Part model, mm, in its own coordinate system. A direction names the side the tool comes from. Round coordinates to 2 decimals unless told otherwise and drop trailing zeros. Return JSON: item names as keys, results as strings. Group by question number.
Item 1: Two-plate mould, pull along Y, no slides. Class faces 1 (the face through (0, 0, 0)), 2 (the face through (-1.625, 5.99, 12.166)), 3 (the face through (-6.73, 14.59, 13.97)), 4 (the face through (-3.042, -5.172, 13.944)): released by +Y, released by -Y, zero draft, split by the parting line, or undercut.
Item 2: Tool access for faces 5 (the face through (0, 0, 19)), 6 (the face through (3.042, 5.172, 13.944)), 7 (the face through (-1, 2, 18)): list every direction of +Z, -Z, +X, -X, +Y, -Y with a clear straight run to the whole face (end or side of a thin tool).
Item 3: Drop flat-ended pins along their axis: pin 1 (7.5 mm diameter, centred on y = -1.5, z = 14, fed in from -X); pin 2 (1.2 mm diameter, centred on x = 0.5, y = -0.5, fed in from +Z); pin 3 (1 mm diameter, centred on x = 5.5, z = 9, fed in from -Y); pin 4 (1.5 mm diameter, centred on x = -7.5, z = 26.5, fed in from -Y). Give the stop position or say it passes through.
Item 4: Probe probe 1 along Y at (x, z) = (0, 23.25); probe 2 along Z at (x, y) = (0.5, -0.75); probe 3 along Z at (x, y) = (-3, -1.75). List the from-to ranges inside material, lowest first.
Item 5: Saw through at A-A on x = -3.25. State how many separate pieces and enclosed holes the cut face has, and give its area (3 significant figures).
```python
from build123d import *

# Parameters (mm, degrees)
SKETCH_1_R          = 2.5
EXTRUDE_1_DEPTH     = 10
EXTRUDE_2_DEPTH     = 8
SKETCH_3_R          = 2
EXTRUDE_3_DEPTH     = 1
SKETCH_5_R          = 0.75
CUT_EXTRUDE_1_DEPTH = 15
SKETCH_6_R          = 2.25
EXTRUDE_4_DEPTH     = 10
SKETCH_7_R          = 1.25
CUT_EXTRUDE_2_DEPTH = 22


with BuildPart() as part:
    # 草图1 → 凸台-拉伸1 (new body)
    with BuildSketch(Plane.XY):
        Circle(SKETCH_1_R)
    extrude(amount=EXTRUDE_1_DEPTH)

    # 草图2 → 凸台-拉伸2 (add)
    with BuildSketch(Plane.XY.offset(10)):
        Polygon((6, 3.464101615), (0, 6.92820323), (-6, 3.464101615), (-6, -3.464101615), (0, -6.92820323), (6, -3.464101615), align=None)
    extrude(amount=EXTRUDE_2_DEPTH)

    # 草图3 → 凸台-拉伸3 (add)
    with BuildSketch(Plane.XY.offset(18)):
        Circle(SKETCH_3_R)
    extrude(amount=EXTRUDE_3_DEPTH)

    # 草图4 → 旋转1 (revolve)
    with BuildSketch(Plane(origin=(0, 0, 0), x_dir=(1, 0, 0), z_dir=(0, 1, 0)), mode=Mode.PRIVATE) as revolve_1_sk:
        Polygon((0, -19), (7.5, -19), (7.5, -27), (1.664204883, -31.183358747), (2.5, -34), (0, -34), align=None)
    revolve(revolve_1_sk.sketch.rotate(Axis((0, 0, 19), (0, 0, 1)), 180), axis=Axis((0, 0, 19), (0, 0, 1)))

    # 草图5 → 切除-拉伸1 (cut)
    with BuildSketch(Plane.XY.offset(34)):
        Circle(SKETCH_5_R)
    extrude(amount=-CUT_EXTRUDE_1_DEPTH, mode=Mode.SUBTRACT)

    # 草图6 → 凸台-拉伸4 (add)
    with BuildSketch(Plane(origin=(-3, 5.196152423, 0), x_dir=(0.8660254037844388, 0.49999999999999983, 0), z_dir=(-0.4999999999999998, 0.8660254037844387, 0))):
        with Locations((0, -14)):
            Circle(SKETCH_6_R)
    extrude(amount=EXTRUDE_4_DEPTH)

    # 草图7 → 切除-拉伸2 (cut)
    with BuildSketch(Plane(origin=(-8, 13.856406461, 0), x_dir=(0.8660254037844387, 0.49999999999999994, 0), z_dir=(-0.4999999999999999, 0.8660254037844386, 0))):
        with Locations(Location((0, -14, 0), (0, 0, 180))):
            Circle(SKETCH_7_R)
    extrude(amount=-CUT_EXTRUDE_2_DEPTH, mode=Mode.SUBTRACT)


solid = part.part
```
Filled in:
{
 "1": {"face 1": "zero draft", "face 2": "undercut", "face 3": "released by +Y", "face 4": "released by -Y"},
 "2": {"face 5": "+Z", "face 6": "-Z, +X, +Y", "face 7": "none"},
 "3": {"pin 1": "stops at x = -6", "pin 2": "stops at z = 34", "pin 3": "passes through", "pin 4": "stops at y = -3.27"},
 "4": {"probe 1": "y = -7.5 to -0.75, 0.75 to 7.5", "probe 2": "z = 0 to 12.75, 15.25 to 34", "probe 3": "z = 10 to 18, 19 to 29.89"},
 "5": {"separate pieces": "2", "enclosed holes": "1", "area": "223 mm^2"}
}
